```python
from build123d import *

# Parameters (mm, degrees)
SKETCH1_W           = 65
SKETCH1_H           = 32
SKETCH1_R           = 1.5
BOSS_EXTRUDE1_DEPTH = 1.5
SKETCH2_W           = 14
SKETCH2_H           = 11
BOSS_EXTRUDE2_DEPTH = 4
SKETCH3_W           = 7
SKETCH3_H           = 8
SKETCH3_W_2         = 4
SKETCH3_H_2         = 4
SKETCH3_W_3         = 9
SKETCH3_H_3         = 7.5
BOSS_EXTRUDE3_DEPTH = 3


with BuildPart() as part:
    # Sketch1 → Boss-Extrude1 (new body)
    with BuildSketch(Plane.XY):
        with Locations((32.5, 16)):
            Rectangle(SKETCH1_W, SKETCH1_H)
        with Locations((2.5, 2.5)):
            Circle(SKETCH1_R, mode=Mode.SUBTRACT)
        with Locations((2.5, 29.5)):
            Circle(SKETCH1_R, mode=Mode.SUBTRACT)
        with Locations((62.5, 29.5)):
            Circle(SKETCH1_R, mode=Mode.SUBTRACT)
        with Locations((62.5, 2.5)):
            Circle(SKETCH1_R, mode=Mode.SUBTRACT)
    extrude(amount=BOSS_EXTRUDE1_DEPTH)

    # Sketch2 → Boss-Extrude2 (add)
    with BuildSketch(Plane.XY.offset(1.5)):
        with Locations((14, 5.5)):
            Rectangle(SKETCH2_W, SKETCH2_H)
        with Locations((51, 5.5)):
            Rectangle(SKETCH2_W, SKETCH2_H)
    extrude(amount=BOSS_EXTRUDE2_DEPTH)

    # Sketch3 → Boss-Extrude3 (add)
    with BuildSketch(Plane.XY.offset(1.5)):
        with Locations((61.5, 21)):
            Rectangle(SKETCH3_W, SKETCH3_H)
        with Locations((63, 9.5)):
            Rectangle(SKETCH3_W_2, SKETCH3_H_2)
        with Locations((32.5, 3.75)):
            Rectangle(SKETCH3_W_3, SKETCH3_H_3)
    extrude(amount=BOSS_EXTRUDE3_DEPTH)


solid = part.part
```
Read the model definition and answer for the solid it produces. Units are mm, in the model's axes. A direction names the side the tool comes from. Coordinates: 2 decimals unless noted, no trailing zeros. Write each loop counter-clockwise with the first axis right and the second up, starting at its lowest first coordinate (ties: lowest second). Pieces come first, ordered by that corner, then holes. Notation, with made-up numbers: (39.25, 84) - (46.25, 84) arc R25 ccw to (46.25, 100) - close; hole circle Ø2 at (76, 13). An arc over 180 degrees is marked (long way). Answer as a JSON object with one key per item and string values. Group by question number.
1. A cutting plane is placed at A-A (x = 2.5). Determine the outline of the cut face in (y, z), plus the area to 3 significant figures.
2. Which of the six approach directions +Z, -Z, +X, -X, +Y, -Y give full straight-line access (tool end or side, diameter ignored) to faces 4 (the flat face through (61, 9, 3)), 5 (the flat face through (21, 5, 3)), 6 (the flat face through (63, 7.5, 3)), 7 (the flat face through (58, 21, 3)), 8 (the flat face through (63, 10, 4.5))?
3. The mould has two halves that part along Y. Classify faces 1 (the flat face through (14, 11, 3)), 2 (the flat face through (32, 4, 4.5)), 3 (the cylindrical face through (2.305, 30.987, 0.74)): +Y half, -Y half, draft (parallel to the pull), parting line (faces both ways), or undercut.
4. A cutting plane is placed at B-B (z = 2.9). Determine the outline of the cut face in (x, y), plus the area to 4 significant figures.
5. A cutting plane is placed at C-C (y = 2.5). Determine the outline of the cut face in (x, z).
6. Consider L1, parallel to Y at x = 62.5, z = 0.8; L2, parallel to X at y = 4, z = 1.65; L3, parallel to X at y = 3, z = 4.9. Determine where each line is inside the solid, lowest interval first. Write a range as [from, to].
7. Each of these flat-tipped pins is pushed along its axis until it touches: P1, Ø0.9, axis at y = 3.5, z = 3, coming from the -X side; P2, Ø2, axis at x = 56.5, y = 27, coming from the +Z side; P3, Ø0.9, axis at x = 61.5, z = 3.5, coming from the +Y side. Where does it stop, or does it pass through?
8. A cutting plane is placed at D-D (y = 9). Determine the outline of the cut face in (x, z).
Worked out:
{
 "1": {"outline": "(0, 0) - (1, 0) - (1, 1.5) - (0, 1.5) - close; (4, 0) - (28, 0) - (28, 1.5) - (4, 1.5) - close; (31, 0) - (32, 0) - (32, 1.5) - (31, 1.5) - close", "area": "39.0 mm²"},
 "2": {"face 4": "+Z, -Y", "face 5": "+Z, +Y, -Y", "face 6": "+Z, +X, -Y", "face 7": "+Z, -X, +Y", "face 8": "+Z, +X, +Y, -Y"},
 "3": {"face 1": "+Y half", "face 2": "draft", "face 3": "undercut"},
 "4": {"outline": "(7, 0) - (21, 0) - (21, 11) - (7, 11) - close; (28, 0) - (37, 0) - (37, 7.5) - (28, 7.5) - close; (44, 0) - (58, 0) - (58, 11) - (44, 11) - close; (58, 17) - (65, 17) - (65, 25) - (58, 25) - close; (61, 7.5) - (65, 7.5) - (65, 11.5) - (61, 11.5) - close", "area": "447.5 mm²"},
 "5": {"outline": "(0, 0) - (1, 0) - (1, 1.5) - (0, 1.5) - close; (4, 0) - (61, 0) - (61, 1.5) - (58, 1.5) - (58, 5.5) - (44, 5.5) - (44, 1.5) - (37, 1.5) - (37, 4.5) - (28, 4.5) - (28, 1.5) - (21, 1.5) - (21, 5.5) - (7, 5.5) - (7, 1.5) - (4, 1.5) - close; (64, 0) - (65, 0) - (65, 1.5) - (64, 1.5) - close"},
 "6": {"L1": "y = [0, 1], [4, 28], [31, 32]", "L2": "x = [7, 21], [28, 37], [44, 58]", "L3": "x = [7, 21], [44, 58]"},
 "7": {"P1": "stops at x = 7", "P2": "stops at z = 1.5", "P3": "stops at y = 25"},
 "8": {"outline": "(0, 0) - (65, 0) - (65, 4.5) - (61, 4.5) - (61, 1.5) - (58, 1.5) - (58, 5.5) - (44, 5.5) - (44, 1.5) - (21, 1.5) - (21, 5.5) - (7, 5.5) - (7, 1.5) - (0, 1.5) - close"}
}
